Can you work these out from the drawing? Everything is in mm from the part's minimum corner. A direction names the side the tool comes from. Coordinates: 2 decimals unless noted, no trailing zeros. Write each loop counter-clockwise with the first axis right and the second up, starting at its lowest first coordinate (ties: lowest second). Pieces come first, ordered by that corner, then holes. Notation, with made-up numbers: (25, 62) -> (74, 62) arc R24 ccw to (74, 78) -> close; hole circle Ø5 at (84, -11.75). An arc over 180 degrees is marked (long way). Use a Markdown table: item, result. Add a question column.
Item 1: If I drill on line 1 along Y through (x, z) = (50.5, 18.9); line 2 along Z through (x, y) = (53, 30); line 3 along Y through (x, z) = (28, 10) (1 decimal), over which ranges is the centre line in solid material (lowest first)? Write a range as from..to.
Item 2: Imagine slicing it at B-B, the plane x = 50.5. Write out the boundary of the cut face in (y, z).
Item 3: Will these pins go through, and if not, where does the flat tip stop? pin 1 Ø3.5 at (x, y) = (50.5, 6.5) entering from +Z; pin 2 Ø4 at (y, z) = (47.5, 2) entering from +X; pin 3 Ø6 at (y, z) = (17, 2.5) entering from -X; pin 4 Ø1 at (x, z) = (24, 15) entering from +Y.
Item 4: Imagine slicing it at D-D, the plane z = 3.25. Write out the boundary of the cut face in (x, y), and give its area (3 significant figures).
Item 5: Imagine slicing it at A-A, the plane x = 28.5. Write out the boundary of the cut face in (y, z), and give its area (3 significant figures).
Item 6: On a 3-axis mill with a long thin cutter (end or side, diameter ignored), from which of +Z, -Z, +X, -X, +Y, -Y can I reach the whole of each face in a straight line? I mean the marked faces 1 and 2. Say none if no direction works.
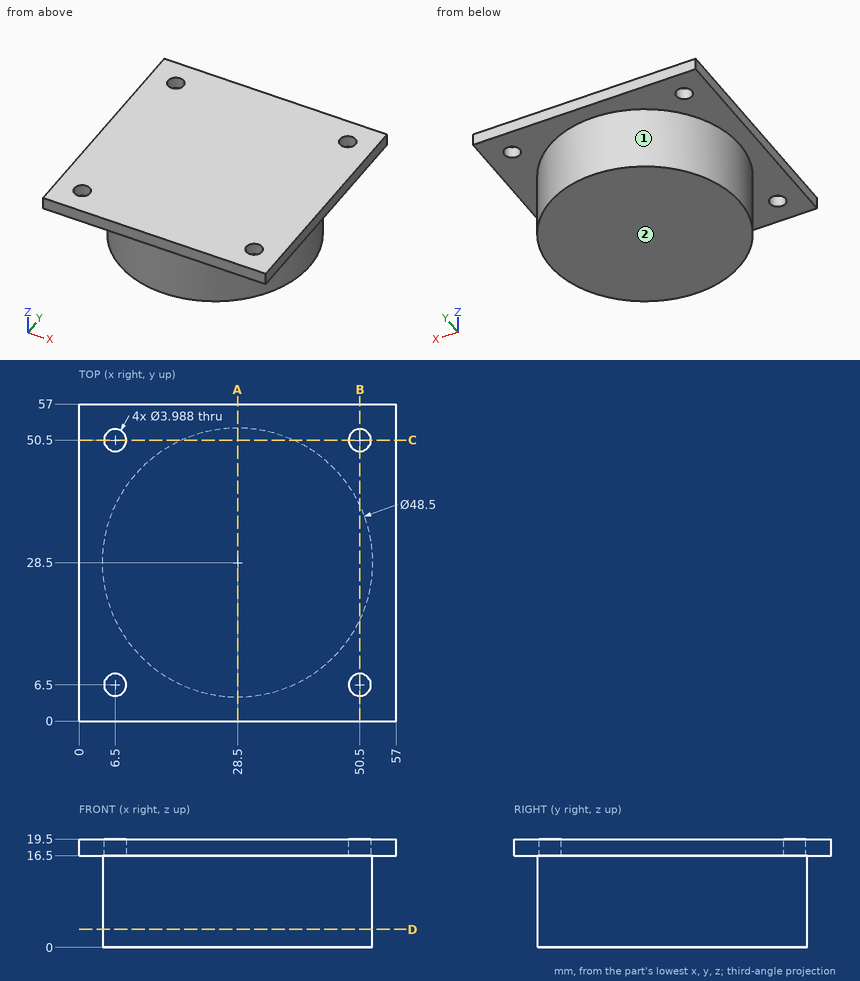
Ans:
| question | item | result |
|---|---|---|
| 1 | line 1 | y = 0..4.51, 8.49..48.51, 52.49..57 |
| 1 | line 2 | z = 16.5..19.5 |
| 1 | line 3 | y = 4.3..52.7 |
| 2 | outline | (0, 16.5) -> (4.51, 16.5) -> (4.51, 19.5) -> (0, 19.5) -> close; (8.49, 16.5) -> (18.3, 16.5) -> (18.3, 0) -> (38.7, 0) -> (38.7, 16.5) -> (48.51, 16.5) -> (48.51, 19.5) -> (8.49, 19.5) -> close; (52.49, 16.5) -> (57, 16.5) -> (57, 19.5) -> (52.49, 19.5) -> close |
| 3 | pin 1 | passes through |
| 3 | pin 2 | stops at x = 45.79 |
| 3 | pin 3 | stops at x = 5.79 |
| 3 | pin 4 | stops at y = 52.42 |
| 4 | outline | circle Ø48.5 at (28.5, 28.5) |
| 4 | area | 1,850 mm^2 |
| 5 | outline | (0, 16.5) -> (4.25, 16.5) -> (4.25, 0) -> (52.75, 0) -> (52.75, 16.5) -> (57, 16.5) -> (57, 19.5) -> (0, 19.5) -> close |
| 5 | area | 971 mm^2 |
| 6 | face 1 | -Z |
| 6 | face 2 | -Z, +X, -X, +Y, -Y |
